from build123d import *

# Parameters (mm, degrees)
F0_R     = 39.651644
F1_DEPTH = 60.96
F2_R     = 28.207671
F3_R     = 36.676793
F4_DEPTH = 40.64
F5_R     = 30.660512


with BuildPart() as f1:
    # F0 (on Top) → F1 (new body)
    with BuildSketch(Plane.XY):
        with Locations((-3.995102, 10.149716)):
            Circle(F0_R)
    extrude(amount=F1_DEPTH)

    # F2
    f2_edges = [f1.edges().sort_by_distance(p)[0] for p in [
        (-43.646746, 10.149716, 60.96),
    ]]
    fillet(f2_edges, radius=F2_R)

    # F3 (on face) → F4 (cut)
    with BuildSketch(Plane(origin=(0, 0, 0), x_dir=(1, 0, 0), z_dir=(0, 0, -1))):
        with Locations((-3.995102, -10.149716)):
            Circle(F3_R)
    extrude(amount=-F4_DEPTH, mode=Mode.SUBTRACT)

    # F5
    f5_edges = [f1.edges().sort_by_distance(p)[0] for p in [
        (-40.671895, 10.149716, 40.64),
    ]]
    fillet(f5_edges, radius=F5_R)


solid = f1.part
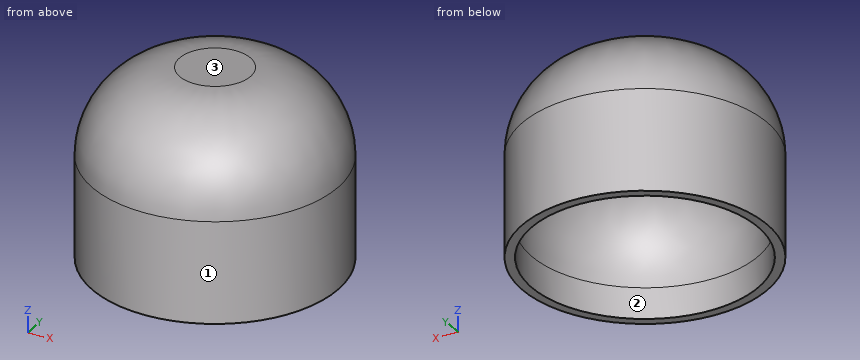
Part model, mm, in its own coordinate system. Face numbers are marked on the shaded views. Coordinates: 2 decimals unless noted, no trailing zeros. Use a Markdown table: item, result. Add a question column.
Q1. Mould opens along Y. For the marked faces 1, 2 and 3 say: +Y half, -Y half, draft (parallel to the pull), parting line (faces both ways), or undercut.
Q2. Probe L1, parallel to X at y = -9, z = 6; L2, parallel to X at y = 38.5, z = 6; L3, parallel to Y at x = 7, z = 10. List the from-to ranges inside material, lowest first.
Q3. Pin check, flat tips, straight feed: P1, Ø10, axis at x = -22.5, y = 1, coming from the -Z side; P2, Ø3.5, axis at x = -4.5, y = 8, coming from the -Z side; P3, Ø4, axis at y = 29.5, z = 32.5, coming from the +X side. Stop position of each tip, or through.
Worked out:
| question | item | result |
|---|---|---|
| 1 | face 1 | parting line |
| 1 | face 2 | undercut |
| 1 | face 3 | draft |
| 2 | L1 | x = -38.72 to -35.28, 27.29 to 30.73 |
| 2 | L2 | x = -31.72 to -27.26, 19.27 to 23.73 |
| 2 | L3 | y = -27.95 to -24.84, 45.14 to 48.25 |
| 3 | P1 | stops at z = 33.53 |
| 3 | P2 | stops at z = 40.64 |
| 3 | P3 | stops at x = 31.66 |
